Here's the drawing with two shaded views (mm, measured from the low corner). I have some questions. A direction names the side the tool comes from. Give positions to 0.01 mm unless a question says otherwise; leave off trailing zeros. Order: outer loops, then holes, each group sorted by start corner. A loop starts at its lowest first (then second) coordinate and runs counter-clockwise, first axis right, second up. Notation, with made-up numbers: M 18,-35.75 L 32,-35.75 A21 cw 32,-11.75 Z; hole C -25,38.25 d9. An arc over 180 degrees is marked long. Use a Markdown table: item, result. Add a question column.
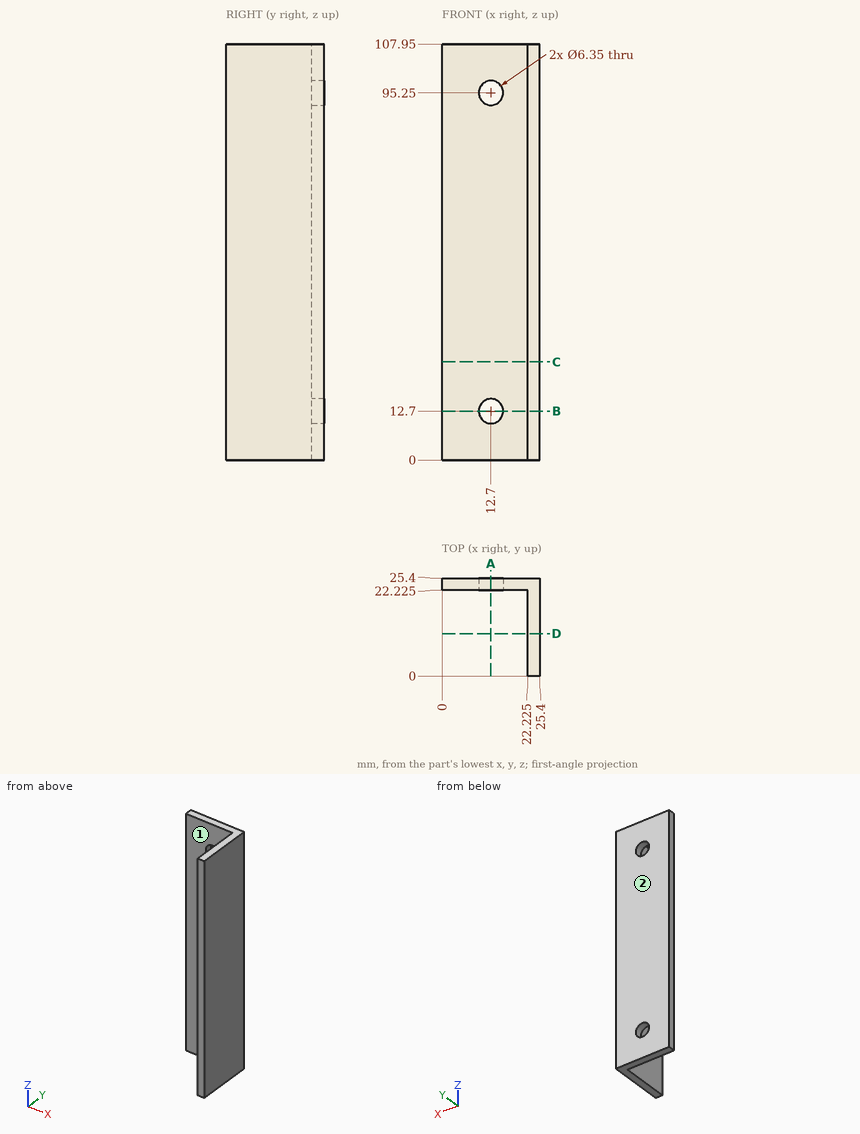
1. Will these pins go through, and if not, where does the flat tip stop? pin 1 (6.5 mm diameter, centred on x = 13.5, z = 37, fed in from -Y) (3 decimals); pin 2 (10 mm diameter, centred on x = 12.7, z = 95.25, fed in from +Y); pin 3 (8 mm diameter, centred on y = 9, z = 26.5, fed in from -X) (3 decimals); pin 4 (12 mm diameter, centred on x = 14.5, y = 12, fed in from +Z).
2. If we section it at D-D, the plane y = 11: List the corners of the cut face in (x, z) for me (3 decimals).
3. If we section it at C-C, the plane z = 25.5: List the corners of the cut face in (x, y) for me (3 decimals), then the cut area to 3 significant figures.
4. If we section it at A-A, the plane x = 12.7: List the corners of the cut face in (y, z) for me (3 decimals).
5. On a 3-axis mill with a long thin cutter (end or side, diameter ignored), from which of +Z, -Z, +X, -X, +Y, -Y can I reach the whole of each face in a straight line? I mean the marked faces 1 and 2. Say none if no direction works.
6. I need wall thicknesses on L1, parallel to X at y = 24.15, z = 12.7 (3 decimals); L2, parallel to X at y = 17, z = 46 (3 decimals). Which ranges of each line are inside material? Lowest first, please. Write a range as [from, to].
7. If we section it at B-B, the plane z = 12.7: List the corners of the cut face in (x, y) for me (3 decimals).
Geometry results:
| question | item | result |
|---|---|---|
| 1 | pin 1 | stops at y = 22.225 |
| 1 | pin 2 | stops at y = 25.4 |
| 1 | pin 3 | stops at x = 22.225 |
| 1 | pin 4 | passes through |
| 2 | outline | M 22.225,0 L 25.4,0 L 25.4,107.95 L 22.225,107.95 Z |
| 3 | outline | M 0,22.225 L 22.225,22.225 L 22.225,0 L 25.4,0 L 25.4,25.4 L 0,25.4 Z |
| 3 | area | 151 mm^2 |
| 4 | outline | M 22.225,0 L 25.4,0 L 25.4,9.525 L 22.225,9.525 Z; M 22.225,15.875 L 25.4,15.875 L 25.4,92.075 L 22.225,92.075 Z; M 22.225,98.425 L 25.4,98.425 L 25.4,107.95 L 22.225,107.95 Z |
| 5 | face 1 | +Z, -Z, -X, -Y |
| 5 | face 2 | +Z, -Z, +X, -X, +Y |
| 6 | L1 | x = [0, 9.525], [15.875, 25.4] |
| 6 | L2 | x = [22.225, 25.4] |
| 7 | outline | M 0,22.225 L 9.525,22.225 L 9.525,25.4 L 0,25.4 Z; M 15.875,22.225 L 22.225,22.225 L 22.225,0 L 25.4,0 L 25.4,25.4 L 15.875,25.4 Z |
